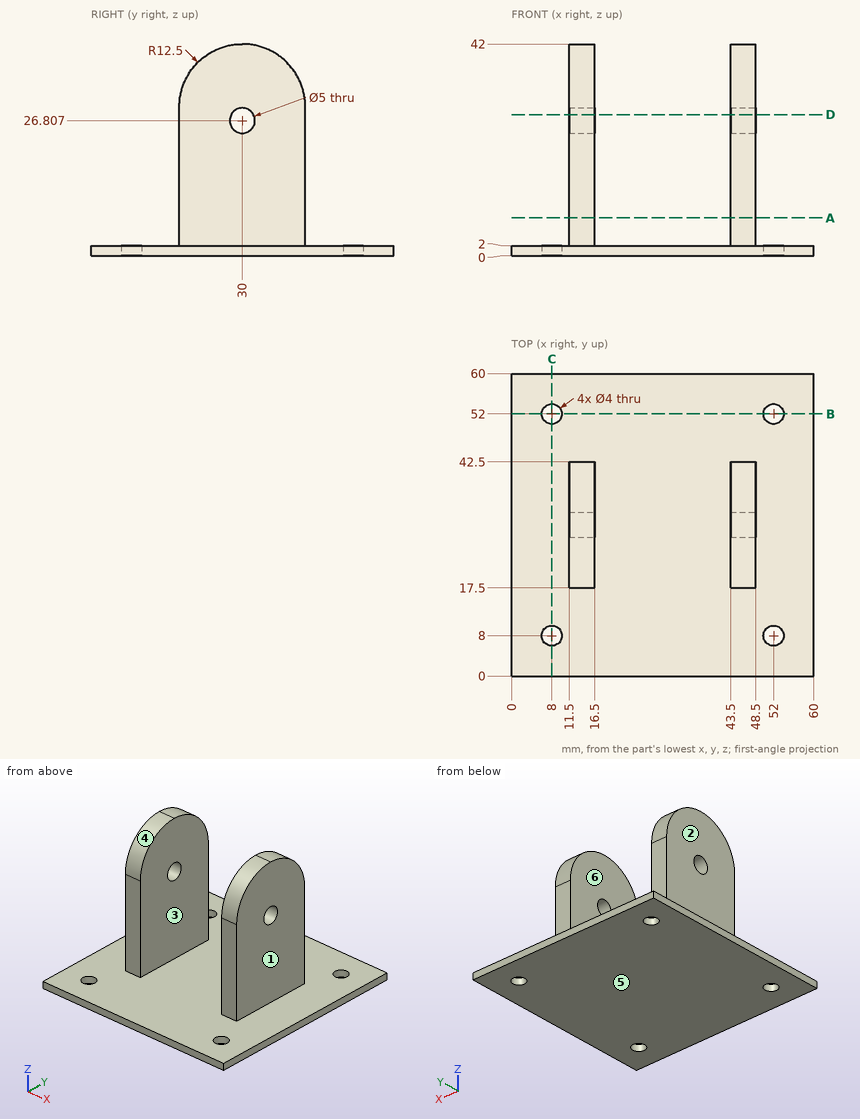
Print and shaded views of the part. All mm, measured from the part's lowest x, y and z. A direction names the side the tool comes from. Coordinates: 2 decimals unless noted, no trailing zeros. Order: outer loops, then holes, each group sorted by start corner. A loop starts at its lowest first (then second) coordinate and runs counter-clockwise, first axis right, second up. Notation, with made-up numbers: (12, 8) - (27, 8) arc R27 ccw to (27, 42) - close; hole circle Ø11 at (79.5, 21.5). An arc over 180 degrees is marked (long way). Return JSON: item names as keys, results as strings. Group by question number.
Item 1: Cut at B-B (y = 52). List the corners of the cut face in (x, z), plus the area to 3 significant figures.
Item 2: Drill centre lines: probe 1 along Y at (x, z) = (52, 1.15); probe 2 along X at (y, z) = (22.5, 29); probe 3 along Z at (x, y) = (46.95, 30). Where is each one in solid material? Low to high. Write a range as from..to.
Item 3: Pull direction X, two halves, no side cores. Call the marked faces 1, 2, 3 and 4: pulls with the +X half, pulls with the -X half, needs draft (parallel to the pull), parting line crosses it, or undercut.
Item 4: Cut at A-A (z = 7.5). List the corners of the cut face in (x, y).
Item 5: Pin check, flat tips, straight feed: pin 1 (12 mm diameter, centred on x = 45, z = 14, fed in from -Y); pin 2 (8 mm diameter, centred on y = 22.5, z = 27, fed in from -X); pin 3 (12 mm diameter, centred on x = 24.5, z = 21, fed in from +Y); pin 4 (4 mm diameter, centred on x = 47, z = 21, fed in from +Y). Stop position of each tip, or through.
Item 6: Which spindle directions (+Z, -Z, +X, -X, +Y, -Y) get a long thin tool onto all of the face, cutting with end or side? Do the marked faces 5 and 6. Say none if no direction does.
Item 7: Cut at D-D (z = 28). List the corners of the cut face in (x, y).
Check values:
{
 "1": {"outline": "(0, 0) - (6, 0) - (6, 2) - (0, 2) - close; (10, 0) - (50, 0) - (50, 2) - (10, 2) - close; (54, 0) - (60, 0) - (60, 2) - (54, 2) - close", "area": "104 mm2"},
 "2": {"probe 1": "y = 0..6, 10..50, 54..60", "probe 2": "x = 11.5..16.5, 43.5..48.5", "probe 3": "z = 0..24.31, 29.31..42"},
 "3": {"face 1": "pulls with the +X half", "face 2": "pulls with the -X half", "face 3": "undercut", "face 4": "needs draft"},
 "4": {"outline": "(11.5, 17.5) - (16.5, 17.5) - (16.5, 42.5) - (11.5, 42.5) - close; (43.5, 17.5) - (48.5, 17.5) - (48.5, 42.5) - (43.5, 42.5) - close"},
 "5": {"pin 1": "stops at y = 17.5", "pin 2": "stops at x = 11.5", "pin 3": "passes through", "pin 4": "stops at y = 42.5"},
 "6": {"face 5": "-Z, +X, -X, +Y, -Y", "face 6": "+Z, +Y, -Y"},
 "7": {"outline": "(11.5, 17.5) - (16.5, 17.5) - (16.5, 27.8) - (11.5, 27.8) - close; (11.5, 32.2) - (16.5, 32.2) - (16.5, 42.5) - (11.5, 42.5) - close; (43.5, 17.5) - (48.5, 17.5) - (48.5, 27.8) - (43.5, 27.8) - close; (43.5, 32.2) - (48.5, 32.2) - (48.5, 42.5) - (43.5, 42.5) - close"}
}
